Drawing for the job (mm, zero at the part's lowest x, y, z). A direction names the side the tool comes from. Coordinates: 2 decimals unless noted, no trailing zeros. Write each loop counter-clockwise with the first axis right and the second up, starting at its lowest first coordinate (ties: lowest second). Pieces come first, ordered by that corner, then holes. Notation, with made-up numbers: M -37.5,-19.75 L -20.5,-19.75 A19 ccw -20.5,-0.75 Z; hole C 87,22.5 d11. An arc over 180 degrees is marked long. Put each result on its own line as item: value. Start each with the question number.
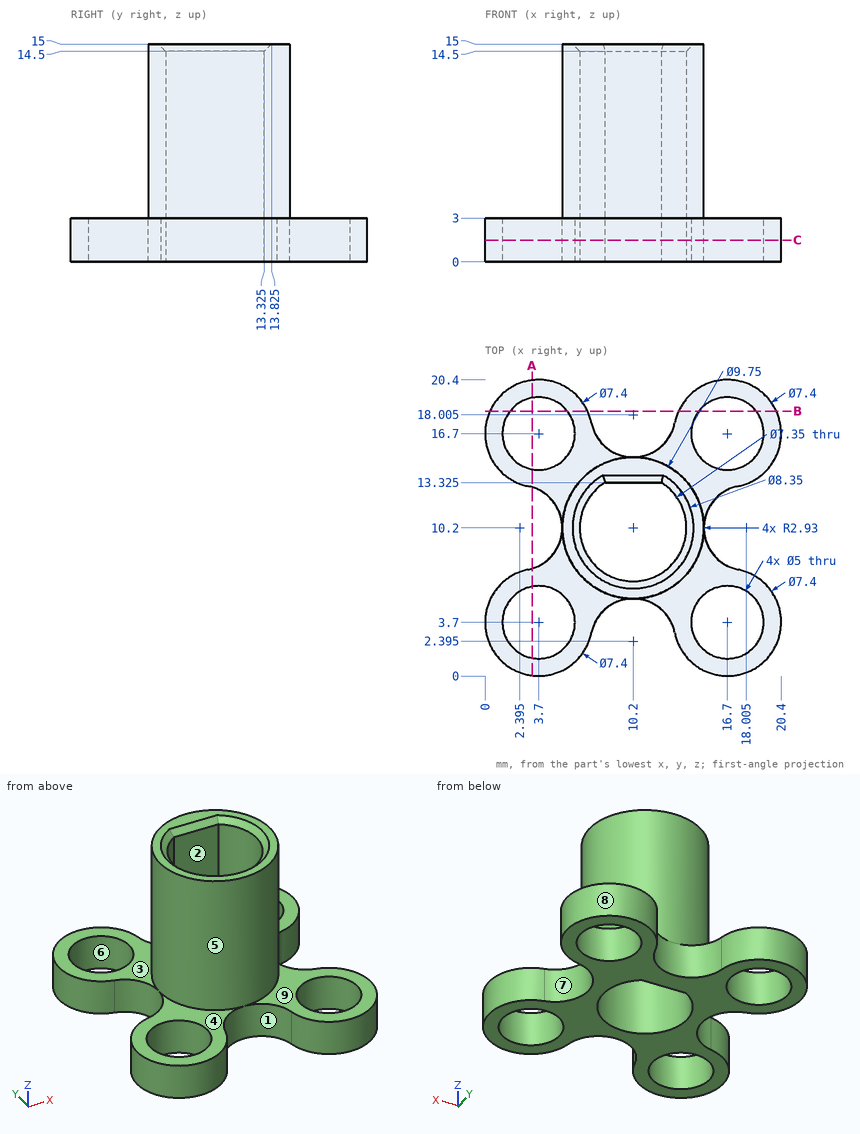
(1) Two-plate mould, pull along X, no slides. Class the marked faces 6, 7, 8 and 9: +X half, -X half, draft (parallel to the pull), parting line (faces both ways), or undercut.
(2) Slice it at B-B, the plane y = 18.25. Write the cut outline in (x, z).
(3) Slice it at A-A, the plane x = 3.25. Write the cut outline in (y, z), then the cut area to 3 significant figures.
(4) Which spindle directions (+Z, -Z, +X, -X, +Y, -Y) get a long thin tool onto all of the face, cutting with end or side? Do the marked faces 1, 2, 3, 4 and 5. Say none if no direction does.
(5) Drop flat-ended pins along their axis: pin 1 (8 mm diameter, centred on x = 8.5, z = 9.5, fed in from +Y) (1 decimal); pin 2 (3 mm diameter, centred on x = 16, y = 14, fed in from +Z); pin 3 (3 mm diameter, centred on x = 11, z = 5.5, fed in from -Y) (1 decimal). Give the stop position or say it passes through.
(6) Drill centre lines: line 1 (Y direction, x = 18.25, z = 2); line 2 (Z direction, x = 6, y = 18.75); line 3 (Y direction, x = 11.25, z = 10.5) (1 decimal). Where is each one in solid material? Low to high. Write a range as [from, to].
(7) Slice it at C-C, the plane z = 1.5. State how many separate pieces and enclosed holes the cut face has.
Result set:
1. face 6: undercut
1. face 7: +X half
1. face 8: undercut
1. face 9: draft
2. outline: M 0.34,0 L 1.74,0 L 1.74,3 L 0.34,3 Z; M 5.66,0 L 7.06,0 L 7.06,3 L 5.66,3 Z; M 13.34,0 L 14.74,0 L 14.74,3 L 13.34,3 Z; M 18.66,0 L 20.06,0 L 20.06,3 L 18.66,3 Z
3. outline: M 0.03,0 L 1.24,0 L 1.24,3 L 0.03,3 Z; M 6.16,0 L 7.4,0 L 7.4,3 L 6.16,3 Z; M 13,0 L 14.24,0 L 14.24,3 L 13,3 Z; M 19.16,0 L 20.37,0 L 20.37,3 L 19.16,3 Z
3. area: 14.7 mm^2
4. face 1: +Z, -Z, -Y
4. face 2: +Z, -Z
4. face 3: +Z, -X, +Y
4. face 4: +Z, -X, -Y
4. face 5: +Z
5. pin 1: stops at y = 15.1
5. pin 2: stops at z = 3
5. pin 3: stops at y = 5.3
6. line 1: y = [0.34, 1.74], [5.66, 7.06], [13.34, 14.74], [18.66, 20.06]
6. line 2: z = [0, 3]
6. line 3: y = [5.4, 6.7], [13.3, 15]
7. separate pieces: 1
7. enclosed holes: 5
